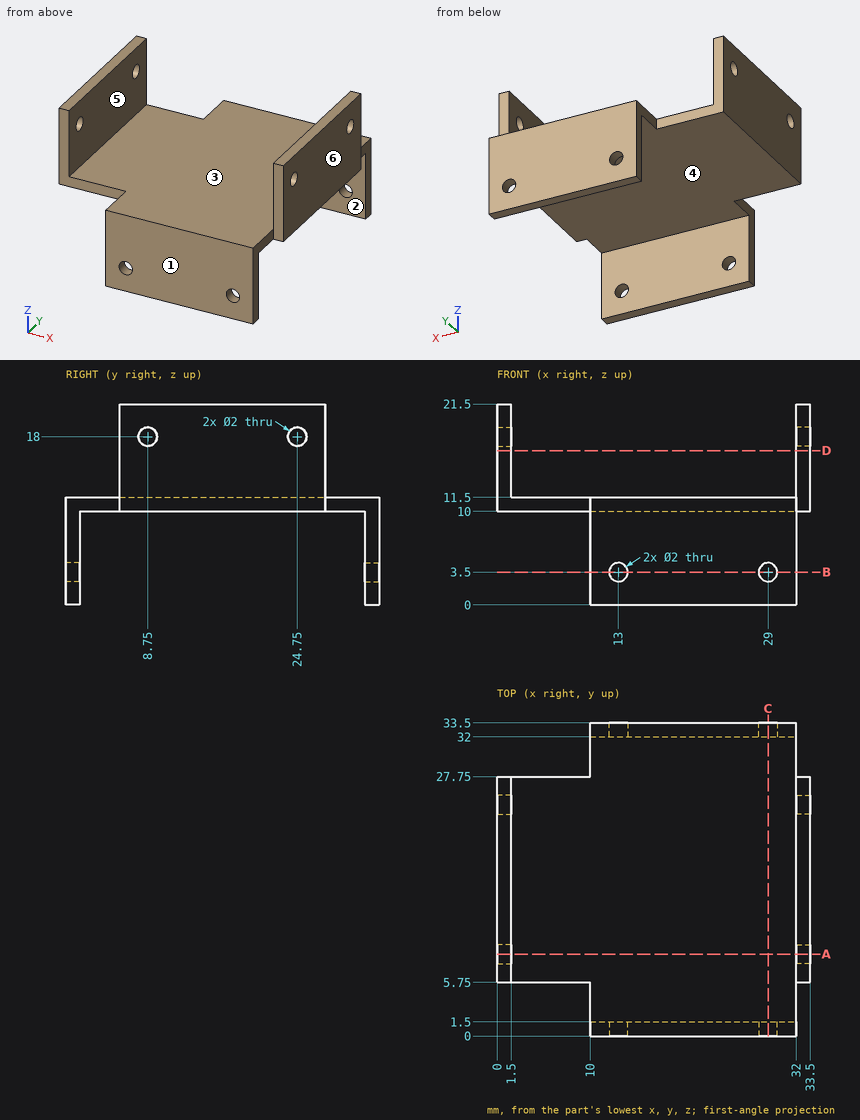
The figure shows three views and two pictorial views of one solid part (mm, origin at its lowest corner). Answer the questions. A direction names the side the tool comes from. Coordinates: 2 decimals unless noted, no trailing zeros. Write each loop counter-clockwise with the first axis right and the second up, starting at its lowest first coordinate (ties: lowest second). Pieces come first, ordered by that corner, then holes. Notation, with made-up numbers: M 29.25,62 L 42.25,62 A15 cw 42.25,75 Z; hole C -19,-19 d10. An arc over 180 degrees is marked long. Answer as CSV lines item,"result". Start each with the question number.
Item 1: Determine the mould class of the marked faces 4, 5 and 6 for opening direction X: released by +X, released by -X, zero draft, split by the parting line, or undercut.
Item 2: Section D-D on z = 16.5 is taken. Write down the section's boundary in (x, y).
Item 3: Consider L1, parallel to Y at x = 33.1, z = 18; L2, parallel to X at y = 15.5, z = 14. Determine where each line is inside the solid, lowest interval first.
Item 4: Section B-B on z = 3.5 is taken. Write down the section's boundary in (x, y), and give its area (3 significant figures).
Item 5: Flat-ended cylindrical pins translate along their axes: P1, Ø3, axis at x = 21, y = 12, coming from the +Z side; P2, Ø4.5, axis at y = 30, z = 6, coming from the -X side; P3, Ø1.7, axis at y = 32, z = 5.5, coming from the +X side. Find the tip coordinate at first contact, or state that the pin passes through.
Item 6: A tool of negligible diameter and unlimited length cuts with its end or side. For the marked faces 1, 2 and 3, from which of +Z, -Z, +X, -X, +Y, -Y can it reach the whole face along a straight path? Write none if from no direction.
Item 7: Section A-A on y = 8.75 is taken. Write down the section's boundary in (x, z), and give its area (4 significant figures).
Item 8: Section C-C on x = 29 is taken. Write down the section's boundary in (y, z), and give its area (4 significant figures).
Checks:
1,face 4,"zero draft"
1,face 5,"undercut"
1,face 6,"released by +X"
2,outline,"M 0,5.75 L 1.5,5.75 L 1.5,27.75 L 0,27.75 Z; M 32,5.75 L 33.5,5.75 L 33.5,27.75 L 32,27.75 Z"
3,L1,"y = 5.75 to 7.75, 9.75 to 23.75, 25.75 to 27.75"
3,L2,"x = 0 to 1.5, 32 to 33.5"
4,outline,"M 10,0 L 12,0 L 12,1.5 L 10,1.5 Z; M 10,32 L 12,32 L 12,33.5 L 10,33.5 Z; M 14,0 L 28,0 L 28,1.5 L 14,1.5 Z; M 14,32 L 28,32 L 28,33.5 L 14,33.5 Z; M 30,0 L 32,0 L 32,1.5 L 30,1.5 Z; M 30,32 L 32,32 L 32,33.5 L 30,33.5 Z"
4,area,"54.0 mm²"
5,P1,"stops at z = 11.5"
5,P2,"stops at x = 10"
5,P3,"stops at x = 32"
6,face 1,"+Z, -Z, +X, -X, -Y"
6,face 2,"-Z, +X, -X"
6,face 3,"+Z, +Y, -Y"
7,outline,"M 0,10 L 33.5,10 L 33.5,17 L 32,17 L 32,11.5 L 1.5,11.5 L 1.5,17 L 0,17 Z; M 0,19 L 1.5,19 L 1.5,21.5 L 0,21.5 Z; M 32,19 L 33.5,19 L 33.5,21.5 L 32,21.5 Z"
7,area,"74.25 mm²"
8,outline,"M 0,0 L 1.5,0 L 1.5,2.5 L 0,2.5 Z; M 0,4.5 L 1.5,4.5 L 1.5,10 L 32,10 L 32,4.5 L 33.5,4.5 L 33.5,11.5 L 0,11.5 Z; M 32,0 L 33.5,0 L 33.5,2.5 L 32,2.5 Z"
8,area,"74.25 mm²"
